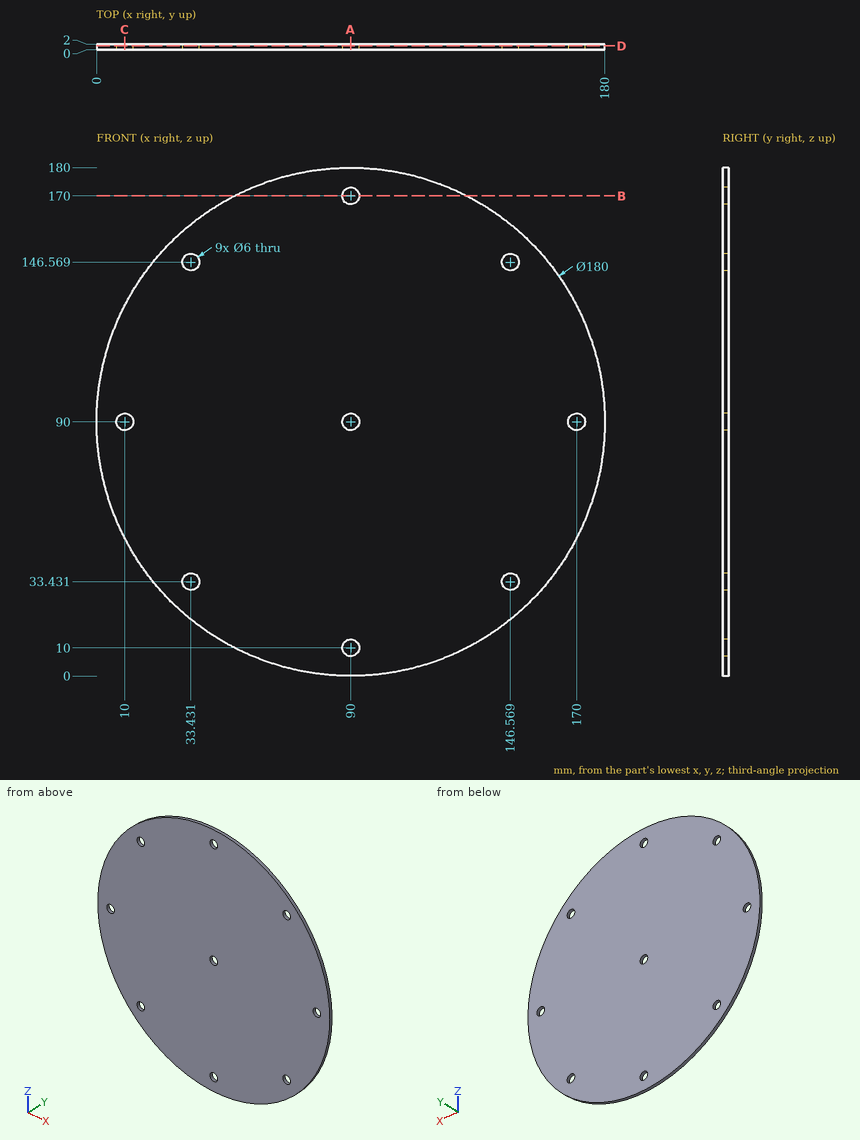
Geometry: see drawing. Coordinates: mm, zero at the bounding-box minimum. Give positions to 0.01 mm unless a question says otherwise; leave off trailing zeros. Order: outer loops, then holes, each group sorted by start corner. A loop starts at its lowest first (then second) coordinate and runs counter-clockwise, first axis right, second up.
Q1. Section D-D on y = 1.35. State how many separate pieces and enclosed holes the cut face has, and give its area (3 significant figures).
Checked values:
separate pieces: 1
enclosed holes: 9
area: 25,200 mm2
Q2. Ray query, probe 1 along X at (y, z) = (1.45, 90); probe 2 along X at (y, z) = (0.95, 92.5) (1 decimal); probe 3 along X at (y, z) = (0.25, 11) (1 decimal). Return the intervals inside material, ascending.
Checked values:
probe 1: x = 0 to 7, 13 to 87, 93 to 167, 173 to 180
probe 2: x = 0 to 8.3, 11.7 to 88.3, 91.7 to 168.3, 171.7 to 180
probe 3: x = 46.9 to 87.2, 92.8 to 133.1
Q3. Section C-C on x = 10. Output: boundary loops of the cut face in (y, z).
Checked values:
outline: (0, 48.77) - (2, 48.77) - (2, 87) - (0, 87) - close; (0, 93) - (2, 93) - (2, 131.23) - (0, 131.23) - close
Q4. Section B-B on z = 170. Output: boundary loops of the cut face in (x, y), and give its area (3 significant figures).
Checked values:
outline: (48.77, 0) - (87, 0) - (87, 2) - (48.77, 2) - close; (93, 0) - (131.23, 0) - (131.23, 2) - (93, 2) - close
area: 153 mm2
Q5. Section A-A on x = 90. Output: boundary loops of the cut face in (y, z), and give its area (3 significant figures).
Checked values:
outline: (0, 0) - (2, 0) - (2, 7) - (0, 7) - close; (0, 13) - (2, 13) - (2, 87) - (0, 87) - close; (0, 93) - (2, 93) - (2, 167) - (0, 167) - close; (0, 173) - (2, 173) - (2, 180) - (0, 180) - close
area: 324 mm2
